CAD build for the part. Positions are in the model's coordinates, mm. Face numbers are marked on the shaded views. A direction names the side the tool comes from. Give positions to 0.01 mm unless a question says otherwise; leave off trailing zeros. Order: outer loops, then holes, each group sorted by start corner. A loop starts at its lowest first (then second) coordinate and runs counter-clockwise, first axis right, second up.
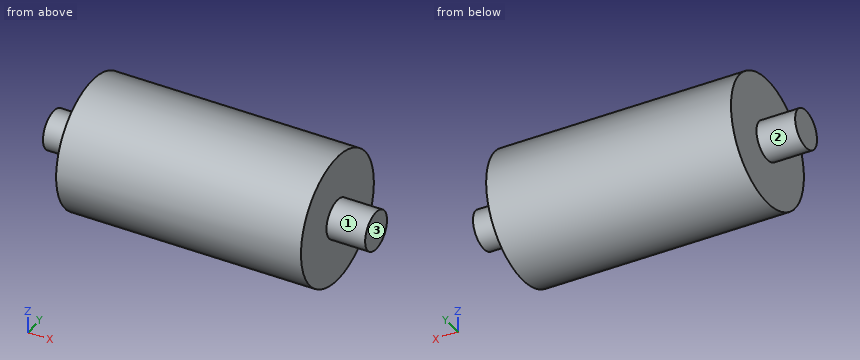
Autodesk Inventor part; units mm, degrees
ref_plane "YZ Plane" through (0, 0, 0) normal (1, 0, 0) x (0, 1, 0)
ref_plane "XZ Plane" through (0, 0, 0) normal (0, 1, 0) x (-1, 0, 0)
ref_plane "XY Plane" through (0, 0, 0) normal (0, 0, 1) x (1, 0, 0)
sketch "Sketch1" plane through (0, 0, 0) normal (1, 0, 0) x (0, 1, 0)
  circle A0 centre (0, 0) radius 10
  dimension "d0" = 20
extrude "Extrusion1" add sketch "Sketch1" along normal blind 50
sketch "Sketch2" plane through (50, 0, 0) normal (1, 0, 0) x (0, 0, -1)
  circle A0 centre (0, 0) radius 10
  circle A1 centre (0, 0) radius 3
  dimension "d3" = 20
  dimension "d4" = 6
extrude "Extrusion2" cut sketch "Sketch2" against normal blind 6
sketch "Sketch3" plane through (0, 0, 0) normal (-1, 0, 0) x (0, 0, 1)
  circle A0 centre (0, 0) radius 10
  circle A1 centre (0, 0) radius 10
  circle A2 centre (0, 0) radius 3
  dimension "d7" = 20
  dimension "d8" = 6
extrude "Extrusion3" cut sketch "Sketch3" against normal blind 6
properties part number "roller"
Item 1: Tool access for the marked faces 1, 2 and 3: list every direction of +Z, -Z, +X, -X, +Y, -Y with a clear straight run to the whole face (end or side of a thin tool).
Item 2: Slice it at D-D (y = -7). Give the cut face in (x, z), and give its area (3 significant figures).
Item 3: Wall check: L1, parallel to X at y = -7.75, z = 1.25; L2, parallel to Y at x = 43.5, z = 0.25; L3, parallel to Z at x = 8.5, y = -1.5. Give the ranges that are in metal, low to high.
Item 4: Slice it at C-C (x = 17). Give the cut face in (y, z), and give its area (3 significant figures).
Item 5: Slice it at A-A (z = 0). Give the cut face in (x, y), and give its area (3 significant figures).
Item 6: Drop flat-ended pins along their axis: pin 1 Ø1 at (y, z) = (0.5, -7.5) entering from +X; pin 2 Ø10 at (x, y) = (29, 5) entering from -Z; pin 3 Ø4 at (y, z) = (-4, -5) entering from -X; pin 4 Ø5 at (x, z) = (22, 4.5) entering from +Y. Give the stop position or say it passes through.
A:
1. face 1: +X
1. face 2: -X
1. face 3: +Z, -Z, +X, +Y, -Y
2. outline: (6, -7.14) - (44, -7.14) - (44, 7.14) - (6, 7.14) - close
2. area: 543 mm2
3. L1: x = 6 to 44
3. L2: y = -10 to 10
3. L3: z = -9.89 to 9.89
4. outline: circle Ø20 at (0, 0)
4. area: 314 mm2
5. outline: (0, -3) - (6, -3) - (6, -10) - (44, -10) - (44, -3) - (50, -3) - (50, 3) - (44, 3) - (44, 10) - (6, 10) - (6, 3) - (0, 3) - close
5. area: 832 mm2
6. pin 1: stops at x = 44
6. pin 2: stops at z = -10
6. pin 3: stops at x = 6
6. pin 4: stops at y = 9.8
